Autodesk Inventor part; units mm, degrees
ref_plane "YZ Plane" through (0, 0, 0) normal (1, 0, 0) x (0, 1, 0)
ref_plane "XZ Plane" through (0, 0, 0) normal (0, 1, 0) x (-1, 0, 0)
ref_plane "XY Plane" through (0, 0, 0) normal (0, 0, 1) x (1, 0, 0)
sketch "Sketch1" plane through (0, 0, 0) normal (0, 0, 1) x (1, 0, 0)
  line L0 (0, 0) -> (0, 7)
  line L1 (0, 0.1034) -> (0, 4.1034)
  arc A0 (0, 7) -> (0, 1.2068) centre (0, 4.1034) ccw
  dimension "d0" = 7
  dimension "d1" = 4
revolve "Revolution1" add sketch "Sketch1" angle 360 about axis through (0, 0.1034, 0) along (0, 1, 0)
sketch "Sketch2" plane through (0, 0, 0) normal (0, 1, 0) x (-1, 0, 0)
  circle A0 centre (0, 0) radius 3.5
  line L0 (0.9209, 3.3767) -> (3.3847, 0.8908)
  line L1 (3.3847, 0.8908) -> (2.4638, -2.4859)
  line L2 (2.4638, -2.4859) -> (-0.9209, -3.3767)
  line L3 (-0.9209, -3.3767) -> (-3.3847, -0.8908)
  line L4 (-3.3847, -0.8908) -> (-2.4638, 2.4859)
  line L5 (-2.4638, 2.4859) -> (0.9209, 3.3767)
  dimension "d3" = 7
extrude "Extrusion1" add sketch "Sketch2" along normal blind 2 contours L1 L2 L3 L4 L5 L0
fillet "Fillet1" radius 0.5 1 edges at (1.9914, 2, 0)
properties part number "5"
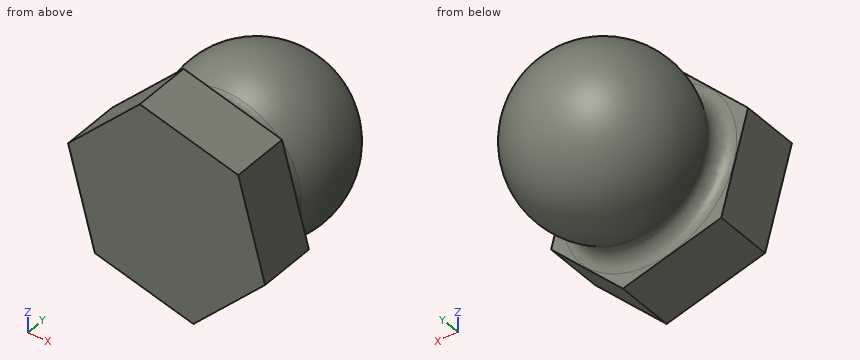
Geometry check sheet. Reference: the model listing, model coordinates, mm. Coordinates: 2 decimals unless noted, no trailing zeros. Write each loop counter-clockwise with the first axis right and the second up, starting at its lowest first coordinate (ties: lowest second). Pieces come first, ordered by that corner, then holes. Notation, with made-up numbers: M 58.25,11 L 105.25,11 A16 cw 105.25,26 Z; hole C -4.5,5.25 d11. An arc over 180 degrees is marked long. One line per item, written item: value. Start each with the question number.
(1) Depth check by flat-ended pin: pin 1 (1 mm diameter, centred on x = -1.5, y = 6, fed in from +Z). Enter the tip coordinate at first touch or a pass-through.
(2) Sectioned sample at C-C, the plane y = 5.5. Enter the section's corners in (x, z).
(3) Sectioned sample at A-A, the plane y = 1.5. Enter the section's corners in (x, z), and give its area (3 significant figures).
(4) Sectioned sample at B-B, the plane y = 4. Enter the section's corners in (x, z), and give its area (3 significant figures).
(5) Scan lines: line 1 along Y through (x, z) = (-2, -2.5); line 2 along Y through (x, z) = (-1.25, 2.25); line 3 along Z through (x, y) = (1, 4). Record each from-to range of solid material in increasing order. Write a range as [from, to].
Filled sheet:
1. pin 1: z = 2.17
2. outline: C 0,0 d5.08
3. outline: M -3.38,0.89 L -2.46,-2.49 L 0.92,-3.38 L 3.38,-0.89 L 2.46,2.49 L -0.92,3.38 Z
3. area: 31.8 mm²
4. outline: C 0,0 d5.79
4. area: 26.3 mm²
5. line 1: [0, 2]
5. line 2: [0, 2.23], [2.77, 5.43]
5. line 3: [-2.72, 2.72]
